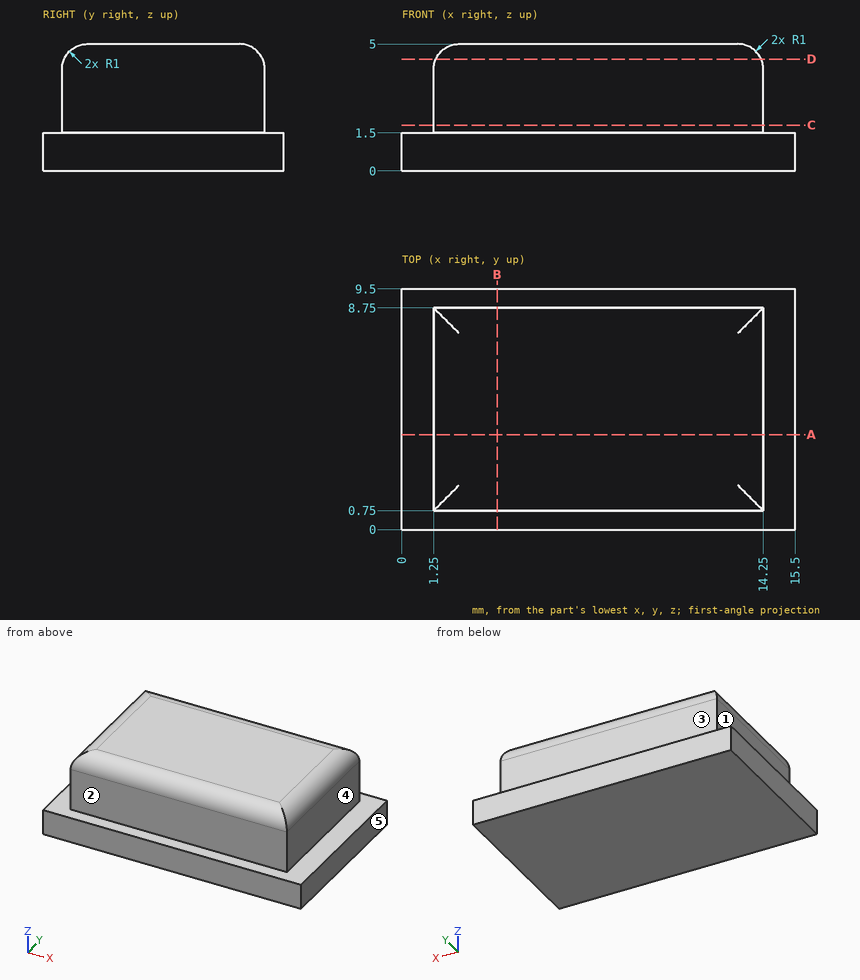
Job drawing, mm, ordinate dimensions from the low corner. One solid piece. A direction names the side the tool comes from. Round coordinates to 2 decimals unless told otherwise and drop trailing zeros. Loops run counter-clockwise (first coordinate to the right, second up) from the corner with the lowest first, then second, coordinate; pieces in that order, holes last. Notation, with made-up numbers: (-12.5, -4.5) -> (44.5, -4.5) arc R13 ccw to (44.5, 15.5) -> close; hole circle Ø5 at (26.25, 53). An arc over 180 degrees is marked (long way). One line per item, written item: value. Start each with the question number.
Q1. Cut at B-B on x = 3.75. List the corners of the cut face in (y, z).
Q2. Drop a flat-ended pin along its axis: pin 1 Ø0.8 at (y, z) = (5, 3.5) entering from -X. Give the stop position or say it passes through.
Q3. Cut at A-A on y = 3.75. List the corners of the cut face in (x, z), plus the area to 3 significant figures.
Q4. Cut at C-C on z = 1.8. List the corners of the cut face in (x, y), plus the area to 3 significant figures.
Q5. Cut at D-D on z = 4.4. List the corners of the cut face in (x, y), plus the area to 3 significant figures.
Q6. Probe line 1 along Y through (x, z) = (4.25, 3.7); line 2 along X through (y, z) = (5.25, 2.75); line 3 along Z through (x, y) = (5, 0.5). List the from-to ranges inside material, lowest first.
Q7. 3-axis set-ups, long thin cutter, end or side, ignore diameter. For the marked faces 1, 2, 3, 4 and 5: which of +Z, -Z, +X, -X, +Y, -Y reach the whole face in a straight line?
Computed:
1. outline: (0, 0) -> (9.5, 0) -> (9.5, 1.5) -> (8.75, 1.5) -> (8.75, 4) arc R1 ccw to (7.75, 5) -> (1.75, 5) arc R1 ccw to (0.75, 4) -> (0.75, 1.5) -> (0, 1.5) -> close
2. pin 1: x = 1.25
3. outline: (0, 0) -> (15.5, 0) -> (15.5, 1.5) -> (14.25, 1.5) -> (14.25, 4) arc R1 ccw to (13.25, 5) -> (2.25, 5) arc R1 ccw to (1.25, 4) -> (1.25, 1.5) -> (0, 1.5) -> close
3. area: 68.3 mm²
4. outline: (1.25, 0.75) -> (14.25, 0.75) -> (14.25, 8.75) -> (1.25, 8.75) -> close
4. area: 104 mm²
5. outline: (1.33, 0.83) -> (14.17, 0.83) -> (14.17, 8.67) -> (1.33, 8.67) -> close
5. area: 101 mm²
6. line 1: 0.75 to 8.75
6. line 2: 1.25 to 14.25
6. line 3: 0 to 1.5
7. face 1: +Z, -X, +Y, -Y
7. face 2: +Z, +X, -X, -Y
7. face 3: +Z, +X, -X, +Y
7. face 4: +Z, +X, +Y, -Y
7. face 5: +Z, -Z, +X, +Y, -Y
